```python
from build123d import *

# Parameters (mm, degrees)
F0_W     = 45
F0_H     = 45
F1_DEPTH = 250
F2_R     = 5
F3_W     = 45
F3_H     = 12.5
F4_DEPTH = 45.001
F5_W     = 40
F5_H     = 20
F6_DEPTH = 25
F7_W     = 40
F7_H     = 20
F8_DEPTH = 25


# Not quite as in the source:
# - a pattern or mirror of a feature is missing from the dataset's text; its kind, count and spacing are read off the source's solid


with BuildPart() as f1:
    # F0 (on Right) → F1 (new body, symmetric)
    with BuildSketch(Plane.YZ):
        with Locations((22.5, 22.5)):
            Rectangle(F0_W, F0_H)
    extrude(amount=F1_DEPTH, both=True)

    # F2
    f2_edges = [f1.edges().sort_by_distance(p)[0] for p in [
        (0, 0, 45),
        (0, 45, 45),
        (0, 0, 0),
        (0, 45, 0),
    ]]
    fillet(f2_edges, radius=F2_R)

    # F3 (on face) → F4 (cut, through all)
    with BuildSketch(Plane.XZ):
        with Locations((-227.5, 6.25)):
            Rectangle(F3_W, F3_H)
        with Locations((-227.5, 38.75)):
            Rectangle(F3_W, F3_H)
    f4 = extrude(amount=-F4_DEPTH, mode=Mode.SUBTRACT)

    # F4_copies: F4 across plane
    add(f4.mirror(Plane(origin=(0, 0, 0), x_dir=(0, 0, 1), z_dir=(1, 0, 0))), mode=Mode.SUBTRACT)

    # F5 (on face) → F6 (cut)
    with BuildSketch(Plane(origin=(-250, 0, 0), x_dir=(0, -1, 0), z_dir=(-1, 0, 0))):
        with Locations((150, 22.5)):
            Rectangle(F5_W, F5_H)
    extrude(amount=-F6_DEPTH, mode=Mode.SUBTRACT)

    # F7 (on face) → F8 (cut)
    with BuildSketch(Plane(origin=(0, 0, 0), x_dir=(1, 0, 0), z_dir=(0, 0, -1))):
        with Locations((-80, -22.5)):
            Rectangle(F7_W, F7_H)
    f8 = extrude(amount=-F8_DEPTH, mode=Mode.SUBTRACT)

    # F8_copies: F8 across plane
    add(f8.mirror(Plane(origin=(0, 0, 0), x_dir=(0, 0, 1), z_dir=(1, 0, 0))), mode=Mode.SUBTRACT)


solid = f1.part
```
Read the model definition and answer for the solid it produces. Units are mm, in the model's axes. A direction names the side the tool comes from. Give positions to 0.01 mm unless a question says otherwise; leave off trailing zeros. Order: outer loops, then holes, each group sorted by start corner. A loop starts at its lowest first (then second) coordinate and runs counter-clockwise, first axis right, second up. Notation, with made-up numbers: (60, -6.75) -> (110, -6.75) arc R21 ccw to (110, 21.25) -> close; hole circle Ø2 at (-14, -38.75). An arc over 180 degrees is marked (long way). Write item = value, one per line.
1. A cutting plane is placed at B-B, the plane x = -72. Write down the section's boundary in (y, z), and give its area (3 significant figures).
Numbers:
outline = (0, 5) arc R5 ccw to (5, 0) -> (12.5, 0) -> (12.5, 25) -> (32.5, 25) -> (32.5, 0) -> (40, 0) arc R5 ccw to (45, 5) -> (45, 40) arc R5 ccw to (40, 45) -> (5, 45) arc R5 ccw to (0, 40) -> close
area = 1,500 mm²
2. Straight lines are drawn through the part: line 1 along X through (y, z) = (18, 19); line 2 along Y through (x, z) = (-96, 24.5); line 3 along Y through (x, z) = (-176, 41). For each, find the intervals that lie inside material, in ascending order.
Numbers:
line_1 = -250 to -100, -60 to 60, 100 to 250
line_2 = 0 to 12.5, 32.5 to 45
line_3 = 0.1 to 44.9
3. A cutting plane is placed at A-A, the plane y = 21.5. Write down the section's boundary in (x, z), and give its area (4 significant figures).
Numbers:
outline = (-250, 12.5) -> (-205, 12.5) -> (-205, 0) -> (-100, 0) -> (-100, 25) -> (-60, 25) -> (-60, 0) -> (60, 0) -> (60, 25) -> (100, 25) -> (100, 0) -> (205, 0) -> (205, 12.5) -> (250, 12.5) -> (250, 32.5) -> (205, 32.5) -> (205, 45) -> (-205, 45) -> (-205, 32.5) -> (-250, 32.5) -> close
area = 18,250 mm²
4. Given pin 1 (10 mm diameter, centred on x = -80.5, y = 27, fed in from -Z); pin 2 (6 mm diameter, centred on x = 67, y = 32, fed in from -Z); pin 3 (6 mm diameter, centred on y = 12.5, z = 7.5, fed in from +X); pin 4 (14 mm diameter, centred on y = 20, z = 41, fed in from -X), each flat-ended and moving along its own axis, determine where each tip first touches the part or whether it passes through.
Numbers:
pin_1 = 25
pin_2 = 0
pin_3 = 205
pin_4 = -205
5. For faces 4 (the face through (-228, 22, 32.5)), 5 (the face through (80, 22, 25)), 6 (the face through (205, 22, 39)), determine the directions among +Z, -Z, +X, -X, +Y, -Y from which every point of the face is accessible in a straight line to the end or side of a thin tool.
Numbers:
face_4 = +Z, -X, +Y, -Y
face_5 = -Z
face_6 = +Z, +X, +Y, -Y
6. The mould has two halves that part along X. Classify faces 1 (the face through (-205, 22, 6)), 2 (the face through (-80, 22, 25)), 3 (the face through (4, 45, 22)): +X half, -X half, draft (parallel to the pull), parting line (faces both ways), or undercut.
Numbers:
face_1 = -X half
face_2 = undercut
face_3 = draft
